The model under review builds one solid part; all positions refer to its coordinate system, in mm. A direction names the side the tool comes from. Coordinates: 2 decimals unless noted, no trailing zeros. Use one line per item in the form item = value.
from build123d import *

# Parameters (mm, degrees)
SKETCH3_R          = 1.5
CUT_EXTRUDE1_DEPTH = 3
FILLET1_R          = 10


with BuildPart() as part:
    # Sketch2 → Loft1 section 0
    with BuildSketch(Plane(origin=(0, 70, 0), x_dir=(1, 0, 0), z_dir=(0, 1, 0))):
        with BuildLine():
            Line((-20, -20), (20, -20))
            Line((20, -20), (20, 20))
            Line((20, 20), (-20, 20))
            Line((-20, 20), (-20, -20))
        make_face()
    # Sketch1 → Loft1 section 1
    with BuildSketch(Plane(origin=(0, 0, 0), x_dir=(1, 0, 0), z_dir=(0, 1, 0))):
        with BuildLine():
            Line((-30, -30), (30, -30))
            Line((30, -30), (30, 30))
            Line((30, 30), (-30, 30))
            Line((-30, 30), (-30, -30))
        make_face()
    loft()

    # Sketch3 → Cut-Extrude1 (cut)
    with BuildSketch(Plane.XZ):
        with Locations(Location((0, 0, 0), (0, 0, 270))):
            Circle(SKETCH3_R)
    cut_extrude1 = extrude(amount=-CUT_EXTRUDE1_DEPTH, mode=Mode.SUBTRACT)

    # Mirror1: Cut-Extrude1 across plane
    add(cut_extrude1.mirror(Plane(origin=(0, 35, 0), x_dir=(0, 0, 1), z_dir=(0, -1, 0))), mode=Mode.SUBTRACT)

    # Fillet1
    fillet1_edges = [part.edges().sort_by_distance(p)[0] for p in [
        (-25, 35, -25),
        (25, 35, -25),
        (25, 35, 25),
        (-25, 35, 25),
    ]]
    fillet(fillet1_edges, radius=FILLET1_R)


solid = part.part
Item 1: Tool access review of faces 1 (the face through (0.45, 68.52, -1.43)), 2 (the face through (0, 3, 0)), 3 (the face through (-4, 70, -3)): name each direction out of +Z, -Z, +X, -X, +Y, -Y from which nothing blocks a thin tool from reaching the whole face with its end or side.
Results found:
face_1 = +Y
face_2 = -Y
face_3 = +Z, -Z, +X, -X, +Y
Item 2: Clearance check with flat-ended pins moving along their axes: pin 1 (0.9 mm diameter, centred on x = 0, z = 0, fed in from +Y); pin 2 (4 mm diameter, centred on y = 15, z = 20.5, fed in from +X); pin 3 (5 mm diameter, centred on y = 56.5, z = 15, fed in from -X); pin 4 (1 mm diameter, centred on x = 23.5, z = 18.5, fed in from -Y). State where each tip first meets the part, or that it passes through.
Results found:
pin_1 = 67
pin_2 = 28.02
pin_3 = -22.14
pin_4 = 0
Item 3: Draft analysis for pull direction Z (two halves, no side actions). For faces 4 (the face through (0.45, 1.48, -1.43)), 5 (the face through (-6, 0, -5)), state which applies: released by +Z, released by -Z, zero draft, split by the parting line, or undercut.
Results found:
face_4 = undercut
face_5 = zero draft
Item 4: To check wall thickness, follow L1, parallel to X at y = 69.15, z = 0; L2, parallel to X at y = 0.6, z = 0; L3, parallel to X at y = 42, z = 21. State the ranges of each line that lie inside material, in increasing order. Write a range as from..to.
Results found:
L1 = -20.12..-1.5, 1.5..20.12
L2 = -29.91..-1.5, 1.5..29.91
L3 = -21.22..21.22
